Input: part model. Units: mm. Frame: model coordinates. A direction names the side the tool comes from. Coordinates: 2 decimals unless noted, no trailing zeros. Order: outer loops, then holes, each group sorted by start corner. A loop starts at its lowest first (then second) coordinate and runs counter-clockwise, first axis right, second up. Notation, with made-up numbers: M 29,14 L 76,14 A4 cw 76,19 Z; hole C 89.25,-1 d1. An arc over 180 degrees is marked long. Answer in a Markdown table with one row per item.
from build123d import *

# Parameters (mm, degrees)
SKETCH1_R           = 6.35
BOSS_EXTRUDE1_DEPTH = 95.25
SKETCH2_R           = 5.08
CUT_EXTRUDE1_DEPTH  = 82.55
SKETCH3_R           = 1.905
CUT_EXTRUDE2_DEPTH  = 114.3
CUT_EXTRUDE8_DEPTH  = 7.62
CUT_REVOLVE1_ANGLE  = 75
SKETCH8_R           = 6.35
SKETCH8_R_2         = 6.2992
CUT_EXTRUDE10_DEPTH = 25.4


with BuildPart() as part:
    # Sketch1 → Boss-Extrude1 (new body)
    with BuildSketch(Plane.XY):
        Circle(SKETCH1_R)
    extrude(amount=BOSS_EXTRUDE1_DEPTH)

    # Sketch2 → Cut-Extrude1 (cut)
    with BuildSketch(Plane(origin=(0, 0, 0), x_dir=(-1, 0, 0), z_dir=(0, 0, -1))):
        Circle(SKETCH2_R)
    extrude(amount=-CUT_EXTRUDE1_DEPTH, mode=Mode.SUBTRACT)

    # Sketch3 → Cut-Extrude2 (cut)
    with BuildSketch(Plane.XY.offset(95.25)):
        Circle(SKETCH3_R)
    extrude(amount=-CUT_EXTRUDE2_DEPTH, mode=Mode.SUBTRACT)

    # Sketch5 → Cut-Extrude8 (cut)
    with BuildSketch(Plane.XY.offset(95.25)):
        with BuildLine():
            ThreePointArc((6.35, 0), (6.299388571, 0.800127257), (6.148361062, 1.5875))
            Line((6.148361062, 1.5875), (3.81, 1.5875))
            Line((3.81, 1.5875), (3.81, -1.5875))
            Line((3.81, -1.5875), (6.148361062, -1.5875))
            ThreePointArc((6.148361062, -1.5875), (6.299388571, -0.800127257), (6.35, 0))
        make_face()
        with BuildLine():
            Line((-3.81, 1.5875), (-6.148361062, 1.5875))
            ThreePointArc((-6.148361062, 1.5875), (-6.35, 0), (-6.148361062, -1.5875))
            Line((-6.148361062, -1.5875), (-3.81, -1.5875))
            Line((-3.81, -1.5875), (-3.81, 1.5875))
        make_face()
    extrude(amount=-CUT_EXTRUDE8_DEPTH, mode=Mode.SUBTRACT)

    # Sketch7 → Cut-Revolve1 (revolve, cut)
    with BuildSketch(Plane(origin=(0, 0, 0), x_dir=(1, 0, 0), z_dir=(0, 1, 0))):
        Polygon((6.148361062, -87.63), (3.81, -87.63), (3.81, -90.805), (6.35, -90.805), (6.35, -87.63), align=None)
        Polygon((-3.81, -90.805), (-6.35, -90.805), (-6.35, -87.63), (-6.148361062, -87.63), (-3.81, -87.63), align=None)
    revolve(axis=Axis((0, 0, 0), (0, 0, 1)), revolution_arc=CUT_REVOLVE1_ANGLE, mode=Mode.SUBTRACT)

    # Sketch8 → Cut-Extrude10 (cut)
    with BuildSketch(Plane.XY.offset(95.25)):
        Circle(SKETCH8_R)
        Circle(SKETCH8_R_2, mode=Mode.SUBTRACT)
    extrude(amount=-CUT_EXTRUDE10_DEPTH, mode=Mode.SUBTRACT)


solid = part.part
1) Mould query, pull axis Y, two halves, no side actions, for faces 1 (the face through (-0.41, -1.86, 88.99)), 2 (the face through (2, 5, 0)), 3 (the face through (-1.38, -6.2, 34.44)). Classes: +Y half, -Y half, draft (parallel to the pull), parting line (faces both ways), or undercut.
Resolved:
| item | result |
|---|---|
| face 1 | undercut |
| face 2 | draft |
| face 3 | parting line |
2) Cut plane A-A, the plane x = 0. Output: boundary loops of the cut face in (y, z) (3 decimals).
Resolved:
| item | result |
|---|---|
| outline | M -6.35,0 L -5.08,0 L -5.08,82.55 L -1.905,82.55 L -1.905,95.25 L -6.299,95.25 L -6.299,69.85 L -6.35,69.85 Z; M 1.905,82.55 L 5.08,82.55 L 5.08,0 L 6.35,0 L 6.35,69.85 L 6.299,69.85 L 6.299,95.25 L 1.905,95.25 Z |
3) Contact query for flat-ended pins moving along their axis: pin 1 (2.5 mm diameter, centred on x = 5, z = 93, fed in from -Y); pin 2 (2 mm diameter, centred on y = -2, z = 73, fed in from +X); pin 3 (2 mm diameter, centred on y = -3, z = 43, fed in from +X). Output: stop coordinate, or through.
Resolved:
| item | result |
|---|---|
| pin 1 | stops at y = -5.06 |
| pin 2 | stops at x = 6.22 |
| pin 3 | stops at x = 6.03 |
4) Cut plane B-B, the plane z = 29. Output: boundary loops of the cut face in (x, y).
Resolved:
| item | result |
|---|---|
| outline | C 0,0 d12.7; hole C 0,0 d10.16 |
5) Material intervals for probe 1 along Z at (x, y) = (1.5, 5) (3 decimals); probe 2 along Y at (x, z) = (0, 42.5); probe 3 along Y at (x, z) = (-2.5, 54), sorted ascending.
Resolved:
| item | result |
|---|---|
| probe 1 | z = 0 to 87.63, 90.805 to 95.25 |
| probe 2 | y = -6.35 to -5.08, 5.08 to 6.35 |
| probe 3 | y = -5.84 to -4.42, 4.42 to 5.84 |
6) Reachability of faces 4 (the face through (-3.81, 0, 92)), 5 (the face through (-1.304, -4.866, 89.195)), 6 (the face through (3.81, 0, 92)), 7 (the face through (0.661, 5.037, 40.697)) from +Z, -Z, +X, -X, +Y, -Y: full face, straight path, thin tool, end or side. Return the list, or none.
Resolved:
| item | result |
|---|---|
| face 4 | +Z, -X |
| face 5 | -X |
| face 6 | +Z, +X |
| face 7 | -Z |
